```python
from build123d import *

# Parameters (mm, degrees)
SKETCH_1_R      = 4.75
SKETCH_1_R_2    = 0.75
EXTRUDE_1_DEPTH = 0.5
EXTRUDE_START   = 0.5
SKETCH_1_3_R    = 1.125
EXTRUDE_2_DEPTH = 0.5


with BuildPart() as part:
    # Sketch 1 → Extrude 1 (new body)
    with BuildSketch(Plane(origin=(0, 0, 0), x_dir=(1, 0, 0), z_dir=(0, 1, 0))):
        with Locations(Location((0, 0, 0), (0, 0, 270))):
            Circle(SKETCH_1_R)
        with Locations(Location((0, 0, 0), (0, 0, 270))):
            Circle(SKETCH_1_R_2, mode=Mode.SUBTRACT)
    extrude(amount=-EXTRUDE_1_DEPTH)

    # Sketch 1_3 → Extrude 2 (add)
    # profile 1 of 2: a face of its own
    with BuildSketch(Plane(origin=(0, 0, 0), x_dir=(1, 0, 0), z_dir=(0, 1, 0)).offset(EXTRUDE_START)):
        with BuildLine():
            Line((1.125, -1), (4.643543905, -1))
            ThreePointArc((4.643543905, -1), (4.723310997, -0.502825243), (4.75, 0))
            ThreePointArc((4.75, 0), (4.348345299, 1.911646713), (3.211308145, 3.5))
            Line((3.211308145, 3.5), (1.125, 3.5))
            Line((1.125, 3.5), (1.125, -1))
        make_face()
        with Locations(Location((2.5, 2, 0), (0, 0, 270))):
            Circle(SKETCH_1_3_R, mode=Mode.SUBTRACT)
    # profile 2 of 2: a face of its own
    with BuildSketch(Plane(origin=(0, 0, 0), x_dir=(1, 0, 0), z_dir=(0, 1, 0)).offset(EXTRUDE_START)):
        with BuildLine():
            ThreePointArc((-3.211308145, 3.5), (-4.526276083, 1.440598771), (-4.643543905, -1))
            Line((-4.643543905, -1), (-1.125, -1))
            Line((-1.125, -1), (-1.125, 3.5))
            Line((-1.125, 3.5), (-3.211308145, 3.5))
        make_face()
        with Locations(Location((-2.5, 2, 0), (0, 0, 270))):
            Circle(SKETCH_1_3_R, mode=Mode.SUBTRACT)
    extrude(amount=-EXTRUDE_2_DEPTH)


solid = part.part
```
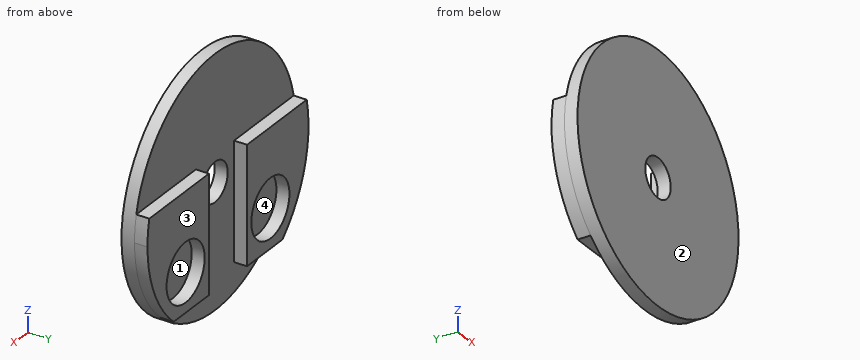
Verification items for the finished model (mm, model axes). Face numbers are marked on the shaded views. A direction names the side the tool comes from. Coordinates: 2 decimals unless noted, no trailing zeros. Loops run counter-clockwise (first coordinate to the right, second up) from the corner with the lowest first, then second, coordinate; pieces in that order, holes last. Notation, with made-up numbers: (85.5, -12) - (111.5, -12) arc R31 ccw to (111.5, 21) - close; hole circle Ø6 at (51.5, 16). An arc over 180 degrees is marked (long way). Answer as a JSON object with one key per item and string values.
(1) Scan lines: line 1 along X through (y, z) = (-0.1, 0); line 2 along X through (y, z) = (0.4, -1.5) (3 decimals); line 3 along X through (y, z) = (0.3, -3) (3 decimals). Record each from-to range of solid material in increasing order.
Response:
{"line 1": "x = -4.75 to -0.75, 0.75 to 4.75", "line 2": "x = -4.507 to -3.508, -1.492 to -1.125, 1.125 to 1.492, 3.508 to 4.507", "line 3": "x = -3.683 to -3.015, -1.985 to -1.125, 1.125 to 1.985, 3.015 to 3.683"}
(2) Go/stop test with flat-tipped pins: pin 1 Ø1.8 at (x, z) = (2.5, -2) entering from +Y; pin 2 Ø0.6 at (y, z) = (0, -2) entering from -X. Record where each tip stops, or that it passes through.
Response:
{"pin 1": "stops at y = 0", "pin 2": "stops at x = -4.44"}
(3) Cross-section at B-B, the plane x = 0. Record the boundary of the cut face in (y, z), then the cut area to 3 significant figures.
Response:
{"outline": "(-0.5, -4.75) - (0, -4.75) - (0, -0.75) - (-0.5, -0.75) - close; (-0.5, 0.75) - (0, 0.75) - (0, 4.75) - (-0.5, 4.75) - close", "area": "4.00 mm²"}
(4) Cross-section at D-D, the plane z = -3. Record the boundary of the cut face in (x, y) (3 decimals).
Response:
{"outline": "(-3.683, -0.5) - (3.683, -0.5) - (3.683, 0.5) - (3.015, 0.5) - (3.015, 0) - (1.985, 0) - (1.985, 0.5) - (1.125, 0.5) - (1.125, 0) - (-1.125, 0) - (-1.125, 0.5) - (-1.985, 0.5) - (-1.985, 0) - (-3.015, 0) - (-3.015, 0.5) - (-3.683, 0.5) - close"}
(5) Mould release check, pull along Z, two halves, no side actions. Record for the marked faces 3 and 4: pulls with the +Z half, pulls with the -Z half, needs draft (parallel to the pull), parting line crosses it, or undercut.
Response:
{"face 3": "needs draft", "face 4": "undercut"}
(6) Access from +Z, -Z, +X, -X, +Y, -Y to the whole of each face (thin tool, end or side, straight path). Record for the marked faces 1 and 2.
Response:
{"face 1": "+Y", "face 2": "+Z, -Z, +X, -X, -Y"}
(7) Cross-section at A-A, the plane y = 0.2. Record the boundary of the cut face in (x, z) (3 decimals), then the cut area to 3 significant figures.
Response:
{"outline": "(-4.644, 1) arc R4.75 ccw to (-3.211, -3.5) - (-1.125, -3.5) - (-1.125, 1) - close; (1.125, -3.5) - (3.211, -3.5) arc R4.75 ccw to (4.644, 1) - (1.125, 1) - close; hole circle Ø2.25 at (-2.5, -2); hole circle Ø2.25 at (2.5, -2)", "area": "21.3 mm²"}
(8) Cross-section at C-C, the plane y = -0.3. Record the boundary of the cut face in (x, z).
Response:
{"outline": "circle Ø9.5 at (0, 0); hole circle Ø1.5 at (0, 0)"}
